The model under review builds one solid part; all positions refer to its coordinate system, in mm. A direction names the side the tool comes from. Give positions to 0.01 mm unless a question says otherwise; leave off trailing zeros. Loops run counter-clockwise (first coordinate to the right, second up) from the corner with the lowest first, then second, coordinate; pieces in that order, holes last. Notation, with made-up numbers: M -23,-16.5 L 9,-16.5 A20 cw 9,4.5 Z; hole C 31.25,-35.75 d4. An arc over 180 degrees is marked long. Return JSON: item names as keys, results as strings.
```python
from build123d import *


with BuildPart() as part:
    # Esquisse1 → Révolution1 (revolve)
    with BuildSketch(Plane.XY, mode=Mode.PRIVATE) as r_volution1_sk:
        with BuildLine():
            Line((200, -60), (200, -180))
            Line((200, -180), (260, -180))
            ThreePointArc((260, -180), (270.606601718, -175.606601718), (275, -165))
            Line((275, -165), (275, -70))
            Line((275, -70), (390, -70))
            Line((390, -70), (390, 0))
            Line((390, 0), (285, 0))
            Line((285, 0), (275, 10))
            Line((275, 10), (275, 370))
            Line((275, 370), (210.606601718, 370))
            Line((210.606601718, 370), (200, 359.393398282))
            Line((200, 359.393398282), (200, 170))
            Line((200, 170), (170, 170))
            Line((170, 170), (170, -60))
            Line((170, -60), (200, -60))
        make_face()
    revolve(r_volution1_sk.sketch.rotate(Axis((0, 425.243902439, 0), (0, -1, 0)), 90), axis=Axis((0, 425.243902439, 0), (0, -1, 0)))


solid = part.part
```
1) Tool access review of faces 1 (the face through (237.3, -34.5, -309.5)), 2 (the face through (-60.075, 263.371, 190.764)), 3 (the face through (-82.6, -116.8, 262.3)): name each direction out of +Z, -Z, +X, -X, +Y, -Y from which nothing blocks a thin tool from reaching the whole face with its end or side.
From the geometry:
{"face 1": "+Y, -Y", "face 2": "+Y", "face 3": "-Y"}
2) Wall thickness on L1, parallel to X at y = 28, z = 0; L2, parallel to X at y = 294, z = 0; L3, parallel to Z at x = -176.5, y = 54.5: over which ranges is each line inside the solid? List them lowest first. Write a range as from..to.
From the geometry:
{"L1": "-275..-170, 170..275", "L2": "-275..-200, 200..275", "L3": "-210.89..210.89"}
3) Insertion check: pin 1 (1 mm diameter, centred on y = 237, z = -12.5, fed in from +X); pin 2 (12 mm diameter, centred on x = 86.5, y = 129.5, fed in from +Z); pin 3 (3 mm diameter, centred on x = 240.5, y = 80, fed in from -Z). Each pin has a flat end and moves straight along its axis. Give the tip position at first contact, or say it passes through.
From the geometry:
{"pin 1": "x = 274.74", "pin 2": "z = 262.95", "pin 3": "z = -136.03"}
4) Consider section C-C on y = 309. Write out the cut boundary in (x, z), then the cut area to 3 significant figures.
From the geometry:
{"outline": "C 0,0 d550; hole C 0,0 d400", "area": "112,000 mm²"}
5) Consider section D-D on y = 72. Write out the cut boundary in (x, z).
From the geometry:
{"outline": "C 0,0 d550; hole C 0,0 d340"}
6) The part is to be moulded in two halves that separate along Z. For faces 4 (the face through (147, -60, 90)), 5 (the face through (81, -70, 265)), 6 (the face through (167.63, 9.51, -218.62)), 7 (the face through (-51.06, 53.39, 162.15)), say which applies: released by +Z, released by -Z, zero draft, split by the parting line, or undercut.
From the geometry:
{"face 4": "undercut", "face 5": "zero draft", "face 6": "split by the parting line", "face 7": "undercut"}
